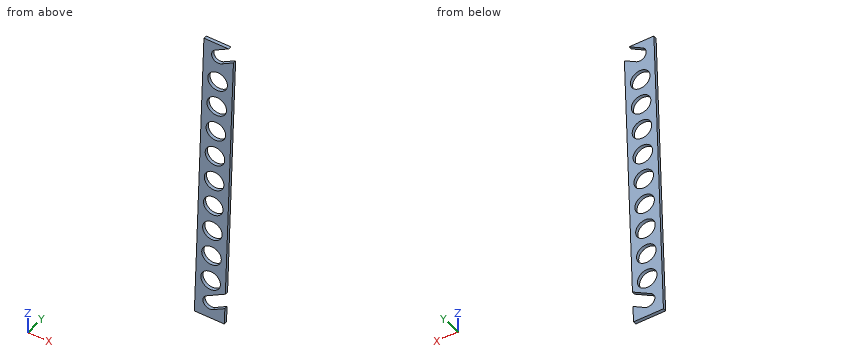
```python
from build123d import *

# Parameters (mm, degrees)
SKETCH1_R           = 4.572
BOSS_EXTRUDE1_DEPTH = 1.5875


with BuildPart() as part:
    # Sketch1 → Boss-Extrude1 (new body)
    with BuildSketch(Plane(origin=(0, 0, 0), x_dir=(1, 0, 0), z_dir=(0, 1, 0))):
        with BuildLine():
            Line((6.776434369, -70.199185368), (-4.764680988, -70.565352679))
            Line((-4.764680988, -70.565352679), (-9.22827802, 70.121395226))
            Line((-9.22827802, 70.121395226), (4.764680988, 70.565352679))
            Line((4.764680988, 70.565352679), (5.016361067, 62.63272534))
            Line((5.016361067, 62.63272534), (-0.466659313, 65.570573089))
            ThreePointArc((-0.466659313, 65.570573089), (-4.833525642, 64.250705768), (-3.51365832, 59.883839439))
            Line((-3.51365832, 59.883839439), (5.252599263, 55.186805992))
            Line((5.252599263, 55.186805992), (9.036951983, -64.09104847))
            Line((9.036951983, -64.09104847), (3.553931604, -61.153200721))
            ThreePointArc((3.553931604, -61.153200721), (-0.812934725, -62.473068042), (0.506932596, -66.839934371))
            Line((0.506932596, -66.839934371), (6.776434369, -70.199185368))
        make_face()
        with Locations(Location((-1.627699267, 51.302954732, 0), (0, 0, 270))):
            Circle(SKETCH1_R, mode=Mode.SUBTRACT)
        with Locations(Location((-1.22077445, 38.477216049, 0), (0, 0, 270))):
            Circle(SKETCH1_R, mode=Mode.SUBTRACT)
        with Locations(Location((-0.813849634, 25.651477366, 0), (0, 0, 270))):
            Circle(SKETCH1_R, mode=Mode.SUBTRACT)
        with Locations(Location((-0.406924817, 12.825738683, 0), (0, 0, 270))):
            Circle(SKETCH1_R, mode=Mode.SUBTRACT)
        with Locations(Location((0, 0, 0), (0, 0, 270))):
            Circle(SKETCH1_R, mode=Mode.SUBTRACT)
        with Locations(Location((0.406924817, -12.825738683, 0), (0, 0, 270))):
            Circle(SKETCH1_R, mode=Mode.SUBTRACT)
        with Locations(Location((0.813849634, -25.651477366, 0), (0, 0, 270))):
            Circle(SKETCH1_R, mode=Mode.SUBTRACT)
        with Locations(Location((1.22077445, -38.477216049, 0), (0, 0, 270))):
            Circle(SKETCH1_R, mode=Mode.SUBTRACT)
        with Locations(Location((1.627699267, -51.302954732, 0), (0, 0, 270))):
            Circle(SKETCH1_R, mode=Mode.SUBTRACT)
    extrude(amount=BOSS_EXTRUDE1_DEPTH)


solid = part.part
```
The listing builds one solid part. Answer for the finished solid, in the listing's coordinates (mm). Give positions to 0.01 mm unless a question says otherwise; leave off trailing zeros. Loops run counter-clockwise (first coordinate to the right, second up) from the corner with the lowest first, then second, coordinate; pieces in that order, holes last. Notation, with made-up numbers: (30, 58.5) - (42, 58.5) arc R23 cw to (42, 71.5) - close; hole circle Ø7 at (66, 38). An arc over 180 degrees is marked (long way). Return JSON: item names as keys, results as strings. Group by question number.
1. Find section C-C (z = 0). Write down the section's boundary in (x, y).
2. Straight lines are drawn through the part: line 1 (X direction, y = 0.35, z = -55); line 2 (X direction, y = 0.65, z = 63); line 3 (X direction, y = 1.25, z = -60). For each, find the intervals that lie inside material, in ascending order. Write a range as [from, to].
3. Find section B-B (y = 1.1). State how many separate pieces and enclosed holes the cut face has, then the cut area to 3 significant figures.
4. Find section A-A (z = -36). Write down the section's boundary in (x, y).
5. Given pin 1 Ø7.5 at (x, z) = (0, 0) entering from +Y (3 decimals); pin 2 Ø10.5 at (x, z) = (0.81, 25.65) entering from +Y, each flat-ended and moving along its own axis, determine where each tip first touches the part or whether it passes through.
Verdict:
{
 "1": {"outline": "(-7, 0) - (-4.57, 0) - (-4.57, 1.59) - (-7, 1.59) - close; (4.57, 0) - (7, 0) - (7, 1.59) - (4.57, 1.59) - close"},
 "2": {"line 1": "x = [-8.75, -4.32], [1.06, 5.26]", "line 2": "x = [-5, -1.04], [7, 9]", "line 3": "x = [-8.91, -3.71]"},
 "3": {"separate pieces": "1", "enclosed holes": "9", "area": "1,240 mm^2"},
 "4": {"outline": "(-8.15, 0) - (-5.06, 0) - (-5.06, 1.59) - (-8.15, 1.59) - close; (2.62, 0) - (5.86, 0) - (5.86, 1.59) - (2.62, 1.59) - close"},
 "5": {"pin 1": "passes through", "pin 2": "stops at y = 1.59"}
}
